Build history of the part. All positions in model axes, mm. Give positions to 0.01 mm unless a question says otherwise; leave off trailing zeros. Loops run counter-clockwise (first coordinate to the right, second up) from the corner with the lowest first, then second, coordinate; pieces in that order, holes last. Notation, with made-up numbers: M 77.5,-4 L 85.5,-4 A34 ccw 85.5,30 Z; hole C -32,46.5 d6. An arc over 180 degrees is marked long. Put each result on its own line as item: value.
```python
from build123d import *

# Parameters (mm, degrees)
SKETCH1_R           = 1.5
BOSS_EXTRUDE1_DEPTH = 2
SKETCH2_R           = 4
CUT_EXTRUDE1_DEPTH  = 136.757961465
SKETCH3_R           = 1.5
CUT_EXTRUDE2_DEPTH  = 10
FILLET1_R           = 10
CUT_EXTRUDE3_DEPTH  = 23
FILLET2_R           = 1


with BuildPart() as part:
    # Sketch1 → Boss-Extrude1 (new body)
    with BuildSketch(Plane(origin=(0, 0, 0), x_dir=(1, 0, 0), z_dir=(0, 1, 0))):
        with BuildLine():
            Line((35.946087305, 32.589224444), (55.068611132, 50.836380863))
            ThreePointArc((55.068611132, 50.836380863), (56.248023483, 52.569022886), (56.613633222, 54.632852189))
            Line((56.613633222, 54.632852189), (54.322448331, 118.551544644))
            ThreePointArc((54.322448331, 118.551544644), (52.732271224, 122.032348819), (49.146545971, 123.369224039))
            Line((49.146545971, 123.369224039), (28.149749669, 122.616587516))
            ThreePointArc((28.149749669, 122.616587516), (24.668945494, 121.026410408), (23.332070273, 117.440685156))
            Line((23.332070273, 117.440685156), (25.181696492, 65.840445524))
            ThreePointArc((25.181696492, 65.840445524), (24.816086753, 63.776616221), (23.636674402, 62.043974198))
            Line((23.636674402, 62.043974198), (5.476247543, 44.714873053))
            ThreePointArc((5.476247543, 44.714873053), (4.296835192, 42.98223103), (3.931225452, 40.918401728))
            Line((3.931225452, 40.918401728), (4.285331317, 31.039677436))
            ThreePointArc((4.285331317, 31.039677436), (3.973516256, 29.113854302), (2.948456097, 27.453952183))
            Line((2.948456097, 27.453952183), (-3.659915658, 20.354208893))
            ThreePointArc((-3.659915658, 20.354208893), (-4.684975817, 18.694306775), (-4.996790878, 16.768483641))
            Line((-4.996790878, 16.768483641), (-4.053596951, -9.544417952))
            Line((-4.053596951, -9.544417952), (-0.700132194, -9.544417952))
            Line((-0.700132194, -9.544417952), (2.299867806, -6.544417952))
            Line((2.299867806, -6.544417952), (18.299867806, -6.544417952))
            Line((18.299867806, -6.544417952), (21.299867806, -9.544417952))
            Line((21.299867806, -9.544417952), (26.299867806, -9.544417952))
            Line((26.299867806, -9.544417952), (28.299867806, -9.544417952))
            Line((28.299867806, -9.544417952), (29.317405641, -9.544417952))
            ThreePointArc((29.317405641, -9.544417952), (31.281555871, -10.276794995), (32.286707076, -12.116342036))
            Line((32.286707076, -12.116342036), (34.27107148, -25.880667111))
            Line((34.27107148, -25.880667111), (37.668448831, -28.421892629))
            Line((37.668448831, -28.421892629), (44.597867771, -27.422897603))
            Line((44.597867771, -27.422897603), (40.206014976, 3.040705467))
            Line((40.206014976, 3.040705467), (35.946087305, 32.589224444))
        make_face()
        with Locations(Location((23.770367042, -5.370271096, 0), (0, 0, 270))):
            Circle(SKETCH1_R, mode=Mode.SUBTRACT)
        with Locations(Location((19.540458754, 3.826449386, 0), (0, 0, 270))):
            Circle(SKETCH1_R, mode=Mode.SUBTRACT)
        with Locations(Location((-1.280541484, -6.226605145, 0), (0, 0, 270))):
            Circle(SKETCH1_R, mode=Mode.SUBTRACT)
        with Locations(Location((3.564149135, 3.664002019, 0), (0, 0, 270))):
            Circle(SKETCH1_R, mode=Mode.SUBTRACT)
    extrude(amount=BOSS_EXTRUDE1_DEPTH)

    # Sketch2 → Cut-Extrude1 (cut, through all)
    with BuildSketch(Plane.XZ):
        with Locations(Location((34.893536441, -107.909402778, 0), (0, 0, 270))):
            Circle(SKETCH2_R)
        with Locations(Location((35.500605714, -90.244703074, 0), (0, 0, 270))):
            Circle(SKETCH2_R)
        with Locations(Location((37.375632996, -51.234404776, 0), (0, 0, 270))):
            Circle(SKETCH2_R)
        with Locations(Location((36.193690526, -72.178757044, 0), (0, 0, 270))):
            Circle(SKETCH2_R)
        with BuildLine():
            Line((9.476681481, -42.336326168), (10.714476932, -7.804732036))
            ThreePointArc((10.714476932, -7.804732036), (12.221884959, -6.401651358), (13.624965636, -7.909059385))
            Line((13.624965636, -7.909059385), (12.387170186, -42.440653517))
            ThreePointArc((12.387170186, -42.440653517), (10.879762159, -43.843734194), (9.476681481, -42.336326168))
        make_face()
        with BuildLine():
            Line((25.946876638, -42.39809035), (27.184672089, -7.866496218))
            ThreePointArc((27.184672089, -7.866496218), (28.736682558, -6.421900022), (30.181278754, -7.973910491))
            Line((30.181278754, -7.973910491), (28.943483303, -42.505504623))
            ThreePointArc((28.943483303, -42.505504623), (27.391472834, -43.950100819), (25.946876638, -42.39809035))
        make_face()
        with BuildLine():
            Line((44.239527936, -115.417065328), (46.189170661, -61.026599384))
            ThreePointArc((46.189170661, -61.026599384), (47.693530634, -59.626355806), (49.093774212, -61.130715778))
            Line((49.093774212, -61.130715778), (47.144131486, -115.521181722))
            ThreePointArc((47.144131486, -115.521181722), (45.639771514, -116.9214253), (44.239527936, -115.417065328))
        make_face()
    extrude(amount=-CUT_EXTRUDE1_DEPTH, mode=Mode.SUBTRACT)

    # Sketch3 → Cut-Extrude2 (cut)
    with BuildSketch(Plane(origin=(0, 2, 0), x_dir=(1, 0, 0), z_dir=(0, 1, 0))):
        with Locations(Location((0, 18.76051869, 0), (0, 0, 270))):
            Circle(SKETCH3_R)
        with Locations(Location((54.054577559, 54.488184987, 0), (0, 0, 270))):
            Circle(SKETCH3_R)
        with Locations(Location((25.943400363, 117.871083174, 0), (0, 0, 270))):
            Circle(SKETCH3_R)
        with Locations(Location((51.146049593, 119.311681239, 0), (0, 0, 270))):
            Circle(SKETCH3_R)
        with Locations(Location((27.939408723, 62.187124606, 0), (0, 0, 270))):
            Circle(SKETCH3_R)
        with Locations(Location((33.240387063, 3.660878573, 0), (0, 0, 270))):
            Circle(SKETCH3_R)
    extrude(amount=-CUT_EXTRUDE2_DEPTH, mode=Mode.SUBTRACT)

    # Fillet1
    fillet1_edges = [part.edges().sort_by_distance(p)[0] for p in [
        (35.946087305, 1, -32.589224444),
    ]]
    fillet(fillet1_edges, radius=FILLET1_R)

    # Sketch4 → Cut-Extrude3 (cut)
    with BuildSketch(Plane.XZ):
        with BuildLine():
            ThreePointArc((36.806162994, 22.440741914), (38.934316746, 23.581659248), (37.215093343, 25.27724223))
            ThreePointArc((37.215093343, 25.27724223), (35.965015311, 24.009735165), (36.806162994, 22.440741914))
        make_face()
        with BuildLine():
            ThreePointArc((34.909100758, 9.281978715), (33.659022726, 8.014471651), (34.500170409, 6.4454784))
            ThreePointArc((34.500170409, 6.4454784), (36.628324161, 7.586395734), (34.909100758, 9.281978715))
        make_face()
    extrude(amount=-CUT_EXTRUDE3_DEPTH, mode=Mode.SUBTRACT)

    # Fillet2
    fillet2_edges = [part.edges().sort_by_distance(p)[0] for p in [
        (21.299867806, 1, 9.544417952),
        (18.299867806, 1, 6.544417952),
        (2.299867806, 1, 6.544417952),
        (-0.700132194, 1, 9.544417952),
        (-4.053596951, 1, 9.544417952),
    ]]
    fillet(fillet2_edges, radius=FILLET2_R)


solid = part.part
```
Q1. Drop flat-ended pins along their axis: pin 1 Ø1 at (x, y) = (-2, 1) entering from +Z; pin 2 Ø1 at (x, y) = (11, 1) entering from +Z. Give the stop position or say it passes through.
Here are the results:
pin 1: z = 9.54
pin 2: z = 6.54
Q2. Mould opens along X. For faces 1 (the cylindrical face through (33.97, 0.99, -93.94)), 2 (the cylindrical face through (37.15, 1.01, -32.24)), 3 (the cylindrical face through (26.01, 1.01, -119.37)), 4 (the cylindrical face through (31.26, 0.99, 10.26)) say: pulls with the +X half, pulls with the -X half, needs draft (parallel to the pull), parting line crosses it, or undercut.
Here are the results:
face 1: undercut
face 2: pulls with the +X half
face 3: undercut
face 4: pulls with the -X half
Q3. Slice it at C-C (y = 1.5). State how many separate pieces and enclosed holes the cut face has, and give its area (3 significant figures).
Here are the results:
separate pieces: 1
enclosed holes: 19
area: 4,260 mm²
Q4. Slice it at D-D (x = 16). List the corners of the cut face in (y, z), and give its area (3 significant figures).
Here are the results:
outline: M 0,-54.76 L 2,-54.76 L 2,6.54 L 0,6.54 Z
area: 123 mm²
Q5. Probe line 1 (X direction, y = 0.5, z = -88); line 2 (X direction, y = 0.95, z = -40); line 3 (Z direction, x = 16.5, y = 1.05). List the from-to ranges inside material, lowest first. Write a range as from..to.
Here are the results:
line 1: 24.39..32.19, 38.81..45.22, 48.13..55.42
line 2: 3.96..9.56, 12.47..26.03, 29.03..43.71
line 3: -55.23..6.54
Q6. Slice it at B-B (z = -90). List the corners of the cut face in (x, y), and give its area (3 significant figures).
Here are the results:
outline: M 24.32,0 L 31.51,0 L 31.51,2 L 24.32,2 Z; M 39.49,0 L 45.15,0 L 45.15,2 L 39.49,2 Z; M 48.06,0 L 55.35,0 L 55.35,2 L 48.06,2 Z
area: 40.3 mm²
Q7. Slice it at A-A (z = -23). List the corners of the cut face in (x, y).
Here are the results:
outline: M -1.2,0 L 10.17,0 L 10.17,2 L -1.2,2 Z; M 13.08,0 L 26.64,0 L 26.64,2 L 13.08,2 Z; M 29.64,0 L 37.33,0 L 37.33,2 L 29.64,2 Z
